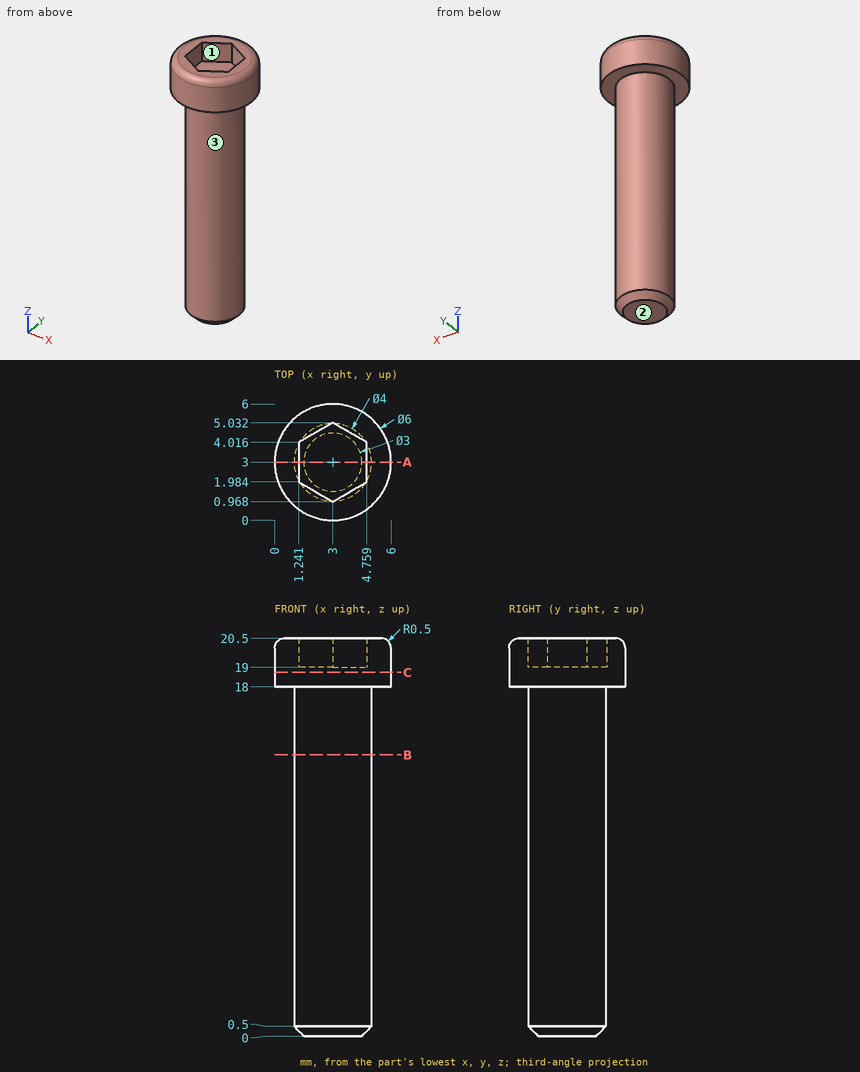
Can you work these out from the drawing? Everything is in mm from the part's minimum corner. Round coordinates to 2 decimals unless told otherwise and drop trailing zeros. Order: outer loops, then holes, each group sorted by start corner. A loop starts at its lowest first (then second) coordinate and runs counter-clockwise, first axis right, second up. Notation, with made-up numbers: (10.25, 44) - (30.25, 44) arc R16 ccw to (30.25, 73) - close; hole circle Ø3 at (41, -21.75). An arc over 180 degrees is marked (long way). Answer in a Markdown table with one row per item.
(1) For P1, Ø2, axis at x = 5, z = 7.5, coming from the +Y side; P2, Ø3, axis at x = 1.5, z = 13.5, coming from the +Y side; P3, Ø1, axis at x = 4.5, z = 16.5, coming from the -Y side, each with a flat end and sliding along its axis, tell me the tip position at first contact or that it passes through.
From the geometry:
| item | result |
|---|---|
| P1 | stops at y = 4.73 |
| P2 | stops at y = 5 |
| P3 | stops at y = 1.27 |
(2) Suppose I cut it at B-B, the plane z = 14.5. Please give me the cut outline in (x, y), plus the area to 3 significant figures.
From the geometry:
| item | result |
|---|---|
| outline | circle Ø4 at (3, 3) |
| area | 12.6 mm2 |
(3) Please list where these lines run through material, in increasing order: L1, parallel to Z at x = 3.5, y = 2; L2, parallel to Z at x = 0.8, y = 2.1; L3, parallel to X at y = 2.25, z = 13.25 (1 decimal). Write a range as from..to.
From the geometry:
| item | result |
|---|---|
| L1 | z = 0..19 |
| L2 | z = 18..20.5 |
| L3 | x = 1.1..4.9 |
(4) If we mould it in two halves opening along X, with no side actions, what happens to the marked faces 1, 2 and 3? For each: released by +X, released by -X, zero draft, split by the parting line, or undercut.
From the geometry:
| item | result |
|---|---|
| face 1 | undercut |
| face 2 | zero draft |
| face 3 | split by the parting line |
(5) Suppose I cut it at C-C, the plane z = 18.75. Please give me the cut outline in (x, y).
From the geometry:
| item | result |
|---|---|
| outline | circle Ø6 at (3, 3) |
(6) Suppose I cut it at A-A, the plane y = 3. Please give me the cut outline in (x, z).
From the geometry:
| item | result |
|---|---|
| outline | (0, 18) - (1, 18) - (1, 0.5) - (1.5, 0) - (4.5, 0) - (5, 0.5) - (5, 18) - (6, 18) - (6, 20) arc R0.5 ccw to (5.5, 20.5) - (4.76, 20.5) - (4.76, 19) - (1.24, 19) - (1.24, 20.5) - (0.5, 20.5) arc R0.5 ccw to (0, 20) - close |
